```python
from build123d import *

# Parameters (mm, degrees)
SKETCH1_W           = 50
SKETCH1_H           = 45
BOSS_EXTRUDE1_DEPTH = 45
SKETCH2_OUTSIDE_W   = 74.472
SKETCH2_OUTSIDE_H   = 69.472
SKETCH2_OUTSIDE_R   = 22.5
CUT_EXTRUDE1_DEPTH  = 10


with BuildPart() as part:
    # Sketch1 → Boss-Extrude1 (new body, symmetric)
    with BuildSketch(Plane(origin=(0, 0, 0), x_dir=(1, 0, 0), z_dir=(0, 1, 0))):
        Rectangle(SKETCH1_W, SKETCH1_H)
    extrude(amount=BOSS_EXTRUDE1_DEPTH, both=True)

    # Sketch2 outside → Cut-Extrude1 (cut, symmetric)
    with BuildSketch(Plane(origin=(0, 45, 0), x_dir=(1, 0, 0), z_dir=(0, 1, 0))):
        Rectangle(SKETCH2_OUTSIDE_W, SKETCH2_OUTSIDE_H)
        Circle(SKETCH2_OUTSIDE_R, mode=Mode.SUBTRACT)
    extrude(amount=CUT_EXTRUDE1_DEPTH, both=True, mode=Mode.SUBTRACT)


solid = part.part
```
CAD build for the part. Positions are in the model's coordinates, mm. A direction names the side the tool comes from. Round coordinates to 2 decimals unless told otherwise and drop trailing zeros. Order: outer loops, then holes, each group sorted by start corner. A loop starts at its lowest first (then second) coordinate and runs counter-clockwise, first axis right, second up.
Item 1: Saw through at A-A on y = 36. Write the cut outline in (x, z).
Item 2: Tool access for faces 1 (the face through (-23, 35, 0)), 2 (the face through (0, -4, 22.5)), 3 (the face through (10.382, 39.93, 19.961)), 4 (the face through (25, -4, 0)), 5 (the face through (23, 35, 0)): list every direction of +Z, -Z, +X, -X, +Y, -Y with a clear straight run to the whole face (end or side of a thin tool).
Item 3: Saw through at C-C on x = -20.5. Write the cut outline in (y, z), then the cut area to 3 significant figures.
Item 4: Probe line 1 along Y through (x, z) = (21, -8.5); line 2 along X through (y, z) = (38, -9); line 3 along Z through (x, y) = (7, 36). List the from-to ranges inside material, lowest first.
Item 5: Saw through at B-B on z = 7. Write the cut outline in (x, y).
Reported:
1. outline: circle Ø45 at (0, 0)
2. face 1: -X, +Y
2. face 2: +Z, +X, -X, +Y, -Y
2. face 3: +Y
2. face 4: +Z, -Z, +X, +Y, -Y
2. face 5: +X, +Y
3. outline: (-45, -22.5) - (35, -22.5) - (35, -9.27) - (45, -9.27) - (45, 9.27) - (35, 9.27) - (35, 22.5) - (-45, 22.5) - close
3. area: 3,790 mm2
4. line 1: y = -45 to 35
4. line 2: x = -20.62 to 20.62
4. line 3: z = -21.38 to 21.38
5. outline: (-25, -45) - (25, -45) - (25, 35) - (21.38, 35) - (21.38, 45) - (-21.38, 45) - (-21.38, 35) - (-25, 35) - close
